Could you check a few things on this model? Use its own coordinates, in mm. Give positions to 0.01 mm unless a question says otherwise; leave off trailing zeros. Loops run counter-clockwise (first coordinate to the right, second up) from the corner with the lowest first, then second, coordinate; pieces in that order, holes last. Notation, with made-up numbers: (77.5, -17.75) -> (114.5, -17.75) arc R14 ccw to (114.5, 9.25) -> close; hole circle Ø3 at (6, 43). An arc over 180 degrees is marked (long way). Write item = value, one per line. Start each with the question number.
1) I want a section at B-B (x = 30). List the corners of the cut face in (y, z) for me.
2) I need wall thicknesses on probe 1 along X at (y, z) = (-14, -286.5); probe 2 along Y at (x, z) = (35, -249.5); probe 3 along Z at (x, y) = (18, -11). Which ranges of each line are inside material? Lowest first, please. Write a range as from..to.
3) I'm going to push a flat-ended pin straight in: pin 1 Ø15 at (x, z) = (23, -257) entering from -Y. Where does the tip first touch, or does it pass through?
4) I want a section at A-A (y = -9.75). List the corners of the cut face in (x, z) for me.
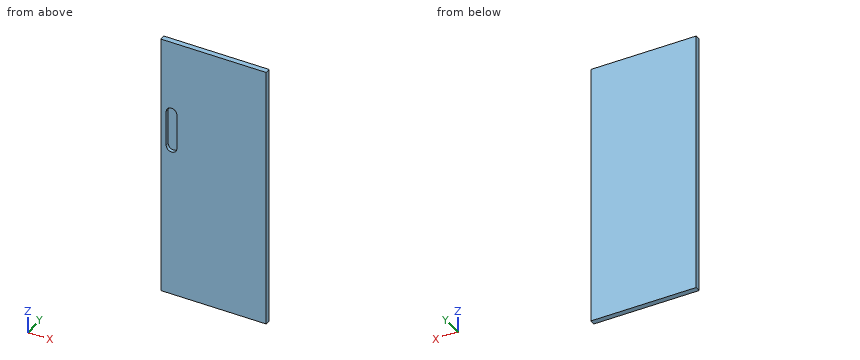
from build123d import *

# Parameters (mm, degrees)
F0_W     = 295
F0_H     = 746
F1_DEPTH = 15
F3_DEPTH = 10


with BuildPart() as f1:
    # F0 (on Front) → F1 (new body)
    with BuildSketch(Plane.XZ):
        with Locations((147.5, -373)):
            Rectangle(F0_W, F0_H)
    extrude(amount=F1_DEPTH)

    # F2 (on face) → F3 (cut)
    with BuildSketch(Plane.XZ.offset(15)):
        with BuildLine():
            ThreePointArc((15, -310), (30, -325), (45, -310))
            ThreePointArc((45, -310), (30, -295), (15, -310))
        make_face()
        with BuildLine():
            Line((45, -310), (45, -210))
            ThreePointArc((45, -210), (30, -225), (15, -210))
            Line((15, -210), (15, -310))
            ThreePointArc((15, -310), (30, -295), (45, -310))
        make_face()
        with BuildLine():
            ThreePointArc((15, -210), (30, -225), (45, -210))
            ThreePointArc((45, -210), (30, -195), (15, -210))
        make_face()
    extrude(amount=-F3_DEPTH, mode=Mode.SUBTRACT)


solid = f1.part
Answer list:
q1.outline = (-15, -746) -> (0, -746) -> (0, 0) -> (-15, 0) -> (-15, -195) -> (-5, -195) -> (-5, -325) -> (-15, -325) -> close
q2.probe_1 = 0..15, 45..295
q2.probe_2 = -5..0
q2.probe_3 = -746..-319, -201..0
q3.pin_1 = -5
q4.outline = (0, -746) -> (295, -746) -> (295, 0) -> (0, 0) -> close; hole (15, -310) arc R15 ccw to (45, -310) -> (45, -210) arc R15 ccw to (15, -210) -> close
